from build123d import *

# Parameters (mm, degrees)
F0_W     = 177.8
F0_H     = 69.85
F1_DEPTH = 81.28
F3_W     = 50.8
F3_H     = 38.1
F4_DEPTH = 69.85
F5_DEPTH = 69.85


with BuildPart() as f1:
    # F0 (on Top) → F1 (new body)
    with BuildSketch(Plane.XY):
        Rectangle(F0_W, F0_H)
    extrude(amount=F1_DEPTH)

    # F3 (on offset) → F4 (cut)
    with BuildSketch(Plane.XZ.offset(34.925)):
        with BuildLine():
            ThreePointArc((-15.970058, 38.1), (-41.370058, 63.5), (-66.770058, 38.1))
            Line((-66.770058, 38.1), (-15.970058, 38.1))
        make_face()
        with Locations((-41.370058, 19.05)):
            Rectangle(F3_W, F3_H)
    extrude(amount=-F4_DEPTH, mode=Mode.SUBTRACT)

    # F3 (on offset) → F5 (cut)
    with BuildSketch(Plane.XZ.offset(34.925)):
        with Locations((41.370058, 19.05)):
            Rectangle(F3_W, F3_H)
        with BuildLine():
            Line((15.970058, 38.1), (66.770058, 38.1))
            ThreePointArc((66.770058, 38.1), (41.370058, 63.5), (15.970058, 38.1))
        make_face()
    extrude(amount=-F5_DEPTH, mode=Mode.SUBTRACT)


solid = f1.part
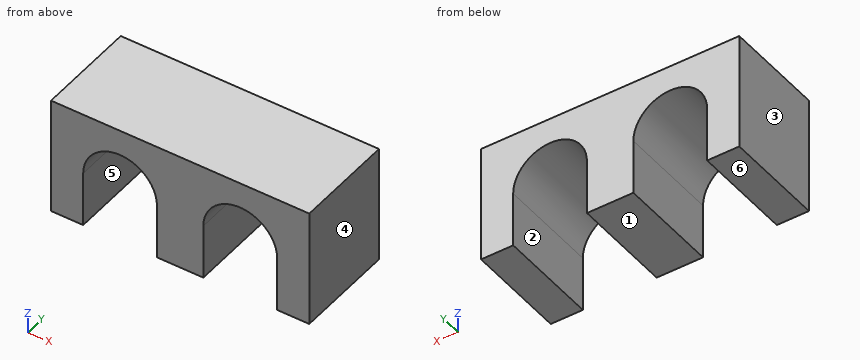
Part model, mm, in its own coordinate system. Face numbers are marked on the shaded views. A direction names the side the tool comes from. Coordinates: 2 decimals unless noted, no trailing zeros. Order: outer loops, then holes, each group sorted by start corner. A loop starts at its lowest first (then second) coordinate and runs counter-clockwise, first axis right, second up. Notation, with made-up numbers: M -16.75,17 L 17.25,17 A30 cw 17.25,43 Z; hole C 88,56 d10. An arc over 180 degrees is marked long. One line per question, with ' | ' between items.
Q1. 3-axis set-ups, long thin cutter, end or side, ignore diameter. For the marked faces 5 and 6: which of +Z, -Z, +X, -X, +Y, -Y reach the whole face in a straight line?
A:
face 5: -Z, +Y, -Y | face 6: -Z, +X, -X, +Y, -Y
Q2. Slice it at A-A (z = 29). Give the cut face in (x, y) (3 decimals), and give its area (3 significant figures).
A:
outline: M -88.9,-34.925 L -66.77,-34.925 L -66.77,34.925 L -88.9,34.925 Z; M -15.97,-34.925 L 15.97,-34.925 L 15.97,34.925 L -15.97,34.925 Z; M 66.77,-34.925 L 88.9,-34.925 L 88.9,34.925 L 66.77,34.925 Z | area: 5,320 mm^2
Q3. Slice it at C-C (x = 33). Give the cut face in (y, z) (3 decimals), and give its area (3 significant figures).
A:
outline: M -34.925,62.081 L 34.925,62.081 L 34.925,81.28 L -34.925,81.28 Z | area: 1,340 mm^2
Q4. Slice it at D-D (x = -30). Give the cut face in (y, z) (3 decimals), and give its area (3 significant figures).
A:
outline: M -34.925,60.813 L 34.925,60.813 L 34.925,81.28 L -34.925,81.28 Z | area: 1,430 mm^2
Q5. Drill centre lines: line 1 (X direction, y = 8, z = 29); line 2 (X direction, y = 29.5, z = 41.5); line 3 (Z direction, x = 40.5, y = -25.5). Where is each one in solid material? Low to high.
A:
line 1: x = -88.9 to -66.77, -15.97 to 15.97, 66.77 to 88.9 | line 2: x = -88.9 to -66.54, -16.2 to 16.2, 66.54 to 88.9 | line 3: z = 63.49 to 81.28
Q6. Two-plate mould, pull along X, no slides. Class the marked faces 1, 2, 3 and 4: +X half, -X half, draft (parallel to the pull), parting line (faces both ways), or undercut.
A:
face 1: draft | face 2: undercut | face 3: -X half | face 4: +X half
Q7. Slice it at B-B (y = 20). Give the cut face in (x, z).
A:
outline: M -88.9,0 L -66.77,0 L -66.77,38.1 A25.4 cw -15.97,38.1 L -15.97,0 L 15.97,0 L 15.97,38.1 A25.4 cw 66.77,38.1 L 66.77,0 L 88.9,0 L 88.9,81.28 L -88.9,81.28 Z
Q8. Pin check, flat tip, straight feed: P1, Ø10, axis at x = -47, y = 21.5, coming from the -Z side. Stop position of the tip, or through.
A:
P1: stops at z = 61.17
